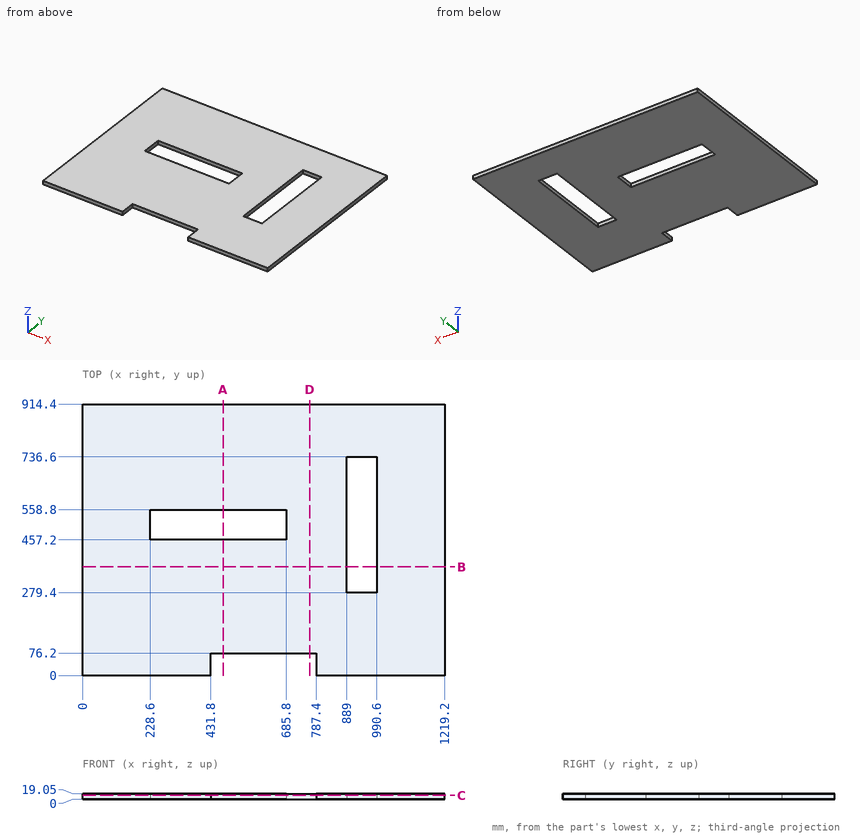
Print and shaded views of the part. All mm, measured from the part's lowest x, y and z. Give positions to 0.01 mm unless a question says otherwise; leave off trailing zeros. Order: outer loops, then holes, each group sorted by start corner. A loop starts at its lowest first (then second) coordinate and runs counter-clockwise, first axis right, second up. Notation, with made-up numbers: (-12, 82) - (29, 82) arc R12 cw to (29, 98) - close; hole circle Ø11 at (29.25, -26.5). An arc over 180 degrees is marked (long way). Use a Markdown table: item, result.
1) Saw through at D-D on x = 764. List the corners of the cut face in (y, z).
Checked values:
| item | result |
|---|---|
| outline | (76.2, 0) - (914.4, 0) - (914.4, 19.05) - (76.2, 19.05) - close |
2) Saw through at A-A on x = 473.5. List the corners of the cut face in (y, z).
Checked values:
| item | result |
|---|---|
| outline | (76.2, 0) - (457.2, 0) - (457.2, 19.05) - (76.2, 19.05) - close; (558.8, 0) - (914.4, 0) - (914.4, 19.05) - (558.8, 19.05) - close |
3) Saw through at C-C on z = 13.75. List the corners of the cut face in (x, y), plus the area to 3 significant figures.
Checked values:
| item | result |
|---|---|
| outline | (0, 0) - (431.8, 0) - (431.8, 76.2) - (787.4, 76.2) - (787.4, 0) - (1219.2, 0) - (1219.2, 914.4) - (0, 914.4) - close; hole (228.6, 457.2) - (685.8, 457.2) - (685.8, 558.8) - (228.6, 558.8) - close; hole (889, 279.4) - (990.6, 279.4) - (990.6, 736.6) - (889, 736.6) - close |
| area | 995,000 mm² |
4) Probe L1, parallel to X at y = 512.5, z = 5; L2, parallel to X at y = 332, z = 7; L3, parallel to Y at x = 957, z = 12. List the from-to ranges inside material, lowest first. Write a range as from..to.
Checked values:
| item | result |
|---|---|
| L1 | 0..228.6, 685.8..889, 990.6..1219.2 |
| L2 | 0..889, 990.6..1219.2 |
| L3 | 0..279.4, 736.6..914.4 |
5) Flat gauge pin, fed straight in: P1, Ø9.5, axis at x = 531, z = 8, coming from the -Y side. Where does the tip first touch, or does it go through?
Checked values:
| item | result |
|---|---|
| P1 | y = 76.2 |
6) Saw through at B-B on y = 366. List the corners of the cut face in (x, z).
Checked values:
| item | result |
|---|---|
| outline | (0, 0) - (889, 0) - (889, 19.05) - (0, 19.05) - close; (990.6, 0) - (1219.2, 0) - (1219.2, 19.05) - (990.6, 19.05) - close |
